Autodesk Inventor part; units mm, degrees
ref_plane "YZ Plane" through (0, 0, 0) normal (1, 0, 0) x (0, 1, 0)
ref_plane "XZ Plane" through (0, 0, 0) normal (0, 1, 0) x (-1, 0, 0)
ref_plane "XY Plane" through (0, 0, 0) normal (0, 0, 1) x (1, 0, 0)
sketch "Sketch1" plane through (0, 0, 0) normal (0, 0, 1) x (1, 0, 0)
  circle A0 centre (0, 0) radius 6.35
  circle A1 centre (0, 0) radius 25.4
  dimension "d0" = 12.7
  dimension "d1" = 50.8
extrude "Extrusion1" add sketch "Sketch1" along normal blind 6.35
sketch "Sketch2" plane through (0, 0, 6.35) normal (0, 0, 1) x (1, 0, 0)
  circle A0 centre (0, 0) radius 6.35
  circle A1 centre (0, 0) radius 12.7
  dimension "d4" = 12.7
  dimension "d5" = 25.4
extrude "Extrusion2" add sketch "Sketch2" along normal blind 12.7
sketch "Sketch3" plane through (0, 0, 19.05) normal (0, 0, 1) x (1, 0, 0)
  circle A0 centre (0, 0) radius 6.35
  circle A1 centre (0, 0) radius 12.7
  line L0 (1.5875, 4.7625) -> (-1.5875, 4.7625)
  line L1 (-1.5875, 4.7625) -> (-1.5875, 7.9375)
  line L2 (-1.5875, 7.9375) -> (1.5875, 7.9375)
  line L3 (1.5875, 7.9375) -> (1.5875, 4.7625)
  line L4 (1.5875, 4.7625) -> (-1.5875, 7.9375) construction
  line L5 (-1.5875, 4.7625) -> (1.5875, 7.9375) construction
  point P0 (0, 6.35)
  dimension "d8" = 3.175
  dimension "d9" = 3.175
extrude "Extrusion3" cut sketch "Sketch3" against normal blind 25.4 contours L3 L0 L1 A0 | A0 L1 L2 L3 picked at (0.1781, 5.2842)
sketch "Sketch4" plane through (0, 0, 6.35) normal (0, 0, 1) x (1, 0, 0)
  circle A0 centre (0, 0) radius 12.7
  circle A1 centre (0, 0) radius 25.4
  circle A2 centre (0, 0) radius 19.05 construction
  circle A3 centre (-19.05, 0) radius 2.413
  circle A4 centre (19.05, 0) radius 2.413
  dimension "d12" = 38.1
  dimension "d13" = 4.826
  dimension "d14" = 4.826
hole "Hole1" at (-19.05, 0, 6.35) at (19.05, 0, 6.35) direction (0, 0, -1) diameter 5.08 end through all
properties part number "Hub Connected to Steel Tubing - 0.5in. Diameter" material "Aluminum 6061"
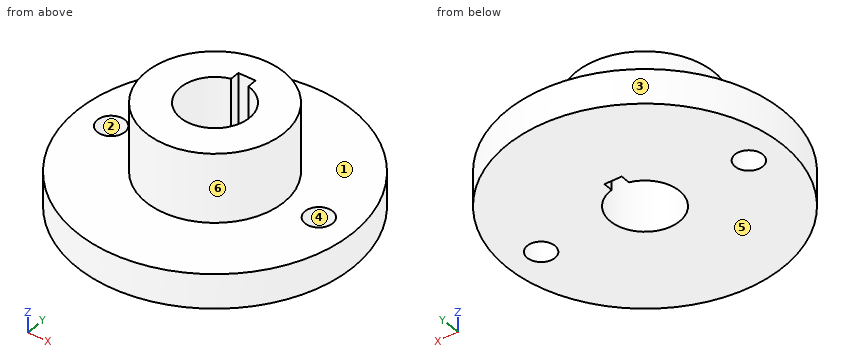
Source: CAD feature listing. Evaluate the final solid. Frame: model axes, mm. Face numbers are marked on the shaded views. A direction names the side the tool comes from. Give positions to 0.01 mm unless a question says otherwise; leave off trailing zeros. Write each loop counter-clockwise with the first axis right and the second up, starting at its lowest first coordinate (ties: lowest second). Pieces come first, ordered by that corner, then holes. Notation, with made-up numbers: M 82.25,-14 L 118.25,-14 A20 cw 118.25,7 Z; hole C 29,38.5 d4. An arc over 180 degrees is marked long. Return JSON: item names as keys, results as strings. Group by question number.
1) Cut plane A-A, the plane x = 0. Output: boundary loops of the cut face in (y, z).
2) Set-up query: the marked faces 5 and 6. Return all of +Z, -Z, +X, -X, +Y, -Y with unobstructed straight access to the full face (end or side cutting, diameter ignored); none if empty.
3) Pin query (flat end, axial travel): P1, Ø6, axis at y = 11, z = 12, coming from the -X side; P2, Ø1, axis at y = 3.5, z = 13.5, coming from the +X side; P3, Ø2.5, axis at x = 0, z = 11.5, coming from the -Y side; P4, Ø10, axis at x = 0, y = 0, coming from the -Z side. Return the tip coordinate at first contact, or that it passes through.
4) Cut plane C-C, the plane z = 4.25. Output: boundary loops of the cut face in (x, y).
5) Cut plane D-D, the plane z = 17.5. Output: boundary loops of the cut face in (x, y), plus the area to 3 significant figures.
6) Pull-direction query (Y, two-part tool) for the marked faces 1, 2, 3 and 4; classes: pulls with the +Y half, pulls with the -Y half, needs draft (parallel to the pull), parting line crosses it, or undercut.
7) Cut plane B-B, the plane y = 0. Output: boundary loops of the cut face in (x, z), plus the area to 3 significant figures.
8) Material intervals for line 1 along Y through (x, z) = (0, 11); line 2 along Z through (x, y) = (-8.5, -22); line 3 along X through (y, z) = (-5, 15.5), sorted ascending. Write a range as [from, to].
Recorded:
{
 "1": {"outline": "M -25.4,0 L -6.35,0 L -6.35,19.05 L -12.7,19.05 L -12.7,6.35 L -25.4,6.35 Z; M 7.94,0 L 25.4,0 L 25.4,6.35 L 12.7,6.35 L 12.7,19.05 L 7.94,19.05 Z"},
 "2": {"face 5": "-Z, +X, -X, +Y, -Y", "face 6": "+Z"},
 "3": {"P1": "stops at x = -9.86", "P2": "stops at x = 12.34", "P3": "stops at y = -12.7", "P4": "passes through"},
 "4": {"outline": "C 0,0 d50.8; hole C -19.05,0 d5.08; hole M -1.59,6.15 A6.35 ccw long 1.59,6.15 L 1.59,7.94 L -1.59,7.94 Z; hole C 19.05,0 d5.08"},
 "5": {"outline": "C 0,0 d25.4; hole M -1.59,6.15 A6.35 ccw long 1.59,6.15 L 1.59,7.94 L -1.59,7.94 Z", "area": "375 mm²"},
 "6": {"face 1": "needs draft", "face 2": "undercut", "face 3": "parting line crosses it", "face 4": "undercut"},
 "7": {"outline": "M -25.4,0 L -21.59,0 L -21.59,6.35 L -25.4,6.35 Z; M -16.51,0 L -6.35,0 L -6.35,19.05 L -12.7,19.05 L -12.7,6.35 L -16.51,6.35 Z; M 6.35,0 L 16.51,0 L 16.51,6.35 L 12.7,6.35 L 12.7,19.05 L 6.35,19.05 Z; M 21.59,0 L 25.4,0 L 25.4,6.35 L 21.59,6.35 Z", "area": "339 mm²"},
 "8": {"line 1": "y = [-12.7, -6.35], [7.94, 12.7]", "line 2": "z = [0, 6.35]", "line 3": "x = [-11.67, -3.91], [3.91, 11.67]"}
}
